Job drawing, mm, ordinate dimensions from the low corner. One solid piece. Round coordinates to 2 decimals unless told otherwise and drop trailing zeros. Write each loop counter-clockwise with the first axis right and the second up, starting at its lowest first coordinate (ties: lowest second). Pieces come first, ordered by that corner, then holes.
1) Drill centre lines: L1, parallel to Z at x = 10.5, y = 3.5; L2, parallel to X at y = 7.75, z = 43; L3, parallel to Z at x = 14.5, y = 7. Where is each one in solid material? Low to high.
2) Pull direction Z, two halves, no side cores. Call the marked faces 1, 2 and 3: +Z half, -Z half, draft (parallel to the pull), parting line (faces both ways), or undercut.
3) Saw through at B-B on z = 26.5. Write the cut outline in (x, y).
4) Saw through at A-A on x = 7.5. Write the cut outline in (y, z), and give its area (3 significant figures).
5) Flat gauge pins, fed straight in: pin 1 (1 mm diameter, centred on y = 4, z = 8.5, fed in from +X); pin 2 (5 mm diameter, centred on x = 5.5, z = 55, fed in from -Y); pin 3 (2 mm diameter, centred on y = 8, z = 35.5, fed in from -X). Where does each tip first touch, or does it go through?
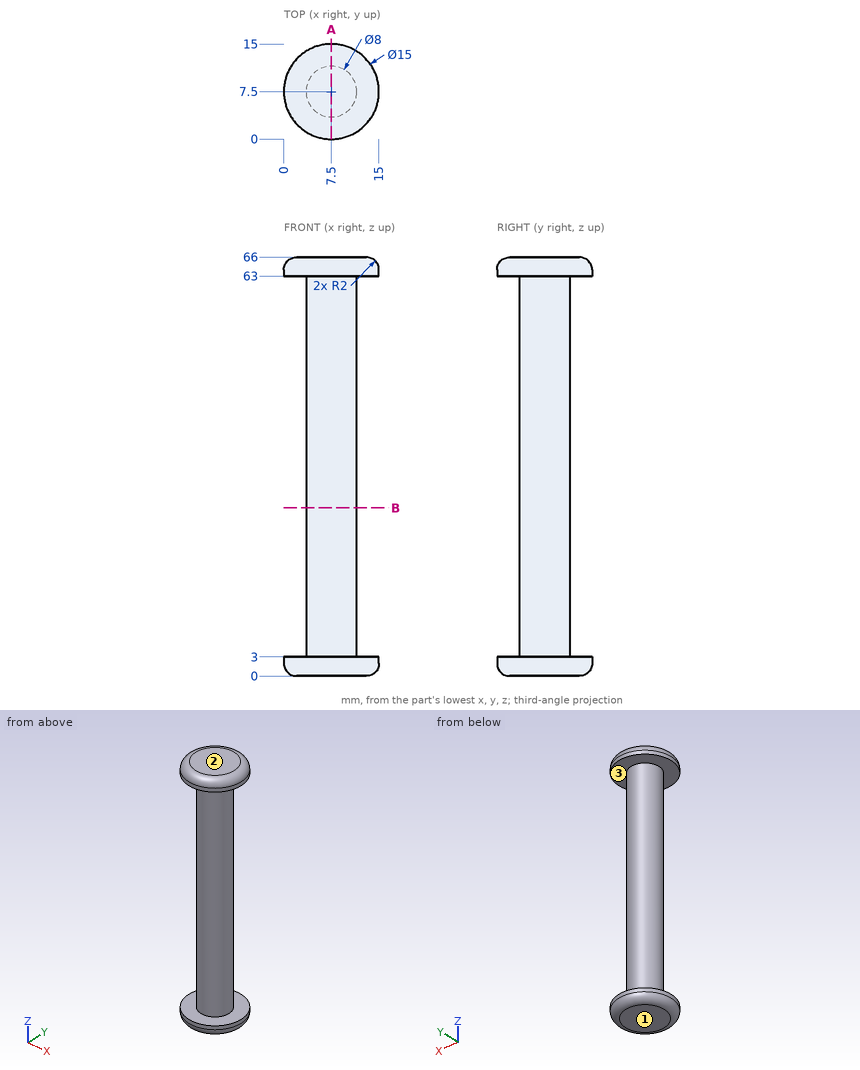
Completed:
1. L1: z = 0 to 3, 63 to 66
1. L2: x = 3.51 to 11.49
1. L3: z = 0.7 to 3, 63 to 65.3
2. face 1: -Z half
2. face 2: +Z half
2. face 3: undercut
3. outline: circle Ø8 at (7.5, 7.5)
4. outline: (0, 2) arc R2 ccw to (2, 0) - (13, 0) arc R2 ccw to (15, 2) - (15, 3) - (11.5, 3) - (11.5, 63) - (15, 63) - (15, 64) arc R2 ccw to (13, 66) - (2, 66) arc R2 ccw to (0, 64) - (0, 63) - (3.5, 63) - (3.5, 3) - (0, 3) - close
4. area: 567 mm2
5. pin 1: stops at x = 10.15
5. pin 2: stops at y = 3.5
5. pin 3: stops at x = 3.5
